from build123d import *

# Parameters (mm, degrees)
F0_W        = 11
F0_H        = 4
F0_W_2      = 10
F1_DEPTH    = 10
F2_DEPTH    = 5
F3_DEPTH    = 15
F5_DEPTH    = 40
F6_T1_DEPTH = 33.0017809158


# Not quite as in the source:
# - a fillet or chamfer that OpenCascade refuses, or shapes differently, is made with other operations: its cross-section is extruded or revolved along the edge and cut away or added


with BuildPart() as f1:
    # F0 (on Front) → F1 (new body)
    with BuildSketch(Plane.XZ):
        Polygon((-5, 4), (5, 4), (20, 4), (20, 7.5), (-20, 7.5), (-20, 4), align=None)
        with BuildLine():
            Line((-5, 0), (-5, 4))
            Line((-5, 4), (-20, 4))
            ThreePointArc((-20, 4), (-17.1715728753, 2.8284271247), (-16, 0))
            Line((-16, 0), (-5, 0))
        make_face()
        with Locations((-10.5, -2)):
            Rectangle(F0_W, F0_H)
        Polygon((16, -4), (5, -4), (-5, -4), (-16, -4), (-16, -7.5), (16, -7.5), align=None)
        with Locations((0, -2)):
            Rectangle(F0_W_2, F0_H)
        with Locations((0, 2)):
            Rectangle(F0_W_2, F0_H)
        with BuildLine():
            Line((20, 4), (5, 4))
            Line((5, 4), (5, 0))
            Line((5, 0), (16, 0))
            ThreePointArc((16, 0), (17.1715728753, 2.8284271247), (20, 4))
        make_face()
        with Locations((10.5, -2)):
            Rectangle(F0_W, F0_H)
    extrude(amount=F1_DEPTH)

    # F0 (on Front) → F2 (join)
    with BuildSketch(Plane.XZ):
        with BuildLine():
            Line((-20, 2), (-20, 4))
            ThreePointArc((-20, 4), (-24, 0), (-20, -4))
            Line((-20, -4), (-20, -2))
            ThreePointArc((-20, -2), (-22, 0), (-20, 2))
        make_face()
        with BuildLine():
            ThreePointArc((-16, 0), (-17.1715728753, 2.8284271247), (-20, 4))
            Line((-20, 4), (-20, 2))
            ThreePointArc((-20, 2), (-18.5857864376, 1.4142135624), (-18, 0))
            ThreePointArc((-18, 0), (-18.5857864376, -1.4142135624), (-20, -2))
            Line((-20, -2), (-20, -4))
            ThreePointArc((-20, -4), (-17.1715728753, -2.8284271247), (-16, 0))
        make_face()
        with BuildLine():
            Line((-16, -4), (-16, 0))
            ThreePointArc((-16, 0), (-17.1715728753, -2.8284271247), (-20, -4))
            Line((-20, -4), (-16, -4))
        make_face()
        with BuildLine():
            ThreePointArc((20, -4), (17.1715728753, -2.8284271247), (16, 0))
            Line((16, 0), (16, -4))
            Line((16, -4), (20, -4))
        make_face()
        with BuildLine():
            Line((20, 2), (20, 4))
            ThreePointArc((20, 4), (17.1715728753, 2.8284271247), (16, 0))
            ThreePointArc((16, 0), (17.1715728753, -2.8284271247), (20, -4))
            Line((20, -4), (20, -2))
            ThreePointArc((20, -2), (18, 0), (20, 2))
        make_face()
        with BuildLine():
            ThreePointArc((24, 0), (22.8284271247, 2.8284271247), (20, 4))
            Line((20, 4), (20, 2))
            ThreePointArc((20, 2), (21.4142135624, 1.4142135624), (22, 0))
            ThreePointArc((22, 0), (21.4142135624, -1.4142135624), (20, -2))
            Line((20, -2), (20, -4))
            ThreePointArc((20, -4), (22.8284271247, -2.8284271247), (24, 0))
        make_face()
    extrude(amount=F2_DEPTH)

    # F0 (on Front) → F3 (join)
    with BuildSketch(Plane.XZ):
        Polygon((16, -4), (5, -4), (-5, -4), (-16, -4), (-16, -7.5), (16, -7.5), align=None)
        with Locations((0, -2)):
            Rectangle(F0_W_2, F0_H)
        with Locations((0, 2)):
            Rectangle(F0_W_2, F0_H)
        Polygon((-5, 4), (5, 4), (20, 4), (20, 7.5), (-20, 7.5), (-20, 4), align=None)
    extrude(amount=F3_DEPTH)

    # F4 (on face) → F5 (cut)
    with BuildSketch(Plane(origin=(-20, 0, 0), x_dir=(0, -1, 0), z_dir=(-1, 0, 0))):
        with BuildLine():
            ThreePointArc((8.5, -5.75), (8.2071067812, -5.0428932188), (7.5, -4.75))
            Line((7.5, -4.75), (7.5, -6.75))
            ThreePointArc((7.5, -6.75), (8.2071067812, -6.4571067812), (8.5, -5.75))
        make_face()
        with BuildLine():
            Line((7.5, -6.75), (7.5, -4.75))
            ThreePointArc((7.5, -4.75), (6.5, -5.75), (7.5, -6.75))
        make_face()
        with BuildLine():
            ThreePointArc((7.5, 6.75), (6.5, 5.75), (7.5, 4.75))
            Line((7.5, 4.75), (7.5, 6.75))
        make_face()
        with BuildLine():
            Line((7.5, 6.75), (7.5, 4.75))
            ThreePointArc((7.5, 4.75), (8.2071067812, 5.0428932188), (8.5, 5.75))
            ThreePointArc((8.5, 5.75), (8.2071067812, 6.4571067812), (7.5, 6.75))
        make_face()
    extrude(amount=-F5_DEPTH, mode=Mode.SUBTRACT)

    # F6: chamfer of 3.5 on 2 edges, made by hand

    # F6_s2 → F6_t1 (cut)
    with BuildSketch(Plane.XZ.offset(-9.0008904579)):
        Polygon((-16, -4), (-12.5, -7.5), (-16, -7.5), align=None)
        Polygon((16, -4), (12.5, -7.5), (16, -7.5), align=None)
    extrude(amount=F6_T1_DEPTH, mode=Mode.SUBTRACT)


solid = f1.part
Input: part model. Units: mm. Frame: model coordinates. A direction names the side the tool comes from. Round coordinates to 2 decimals unless told otherwise and drop trailing zeros. Order: outer loops, then holes, each group sorted by start corner. A loop starts at its lowest first (then second) coordinate and runs counter-clockwise, first axis right, second up. Notation, with made-up numbers: (-9, 0.25) - (6, 0.25) arc R21 cw to (6, 14.25) - close; hole circle Ø3 at (-30.75, -23.5). An arc over 180 degrees is marked (long way). Answer as a JSON object with one key per item and string values. Group by question number.
(1) Cut plane C-C (z = 1). Return loops of the section in (x, y).
(2) Cut plane B-B (y = -11.5). Return loops of the section in (x, z).
(3) Reachability of faces 1 (the face through (-18, -2, -4)), 2 (the face through (-17.203, -7.465, 2.859)), 3 (the face through (18, -5, -1)), 4 (the face through (-13, -12, 4)), 5 (the face through (-20, -7, 7)) from +Z, -Z, +X, -X, +Y, -Y: full face, straight path, thin tool, end or side. Return the list, or none.
(4) Draft query along Z for faces 6 (the face through (-10, -12, -4)), 7 (the face through (15.4, -7.4, -4.6)), 8 (the face through (-16, -7, -2)). Return one class per face: released by +Z, released by -Z, zero draft, split by the parting line, or undercut.
(5) Cut plane A-A (x = 6). Return loops of the section in (y, z), then the cut area to 3 significant figures.
(6) Pin query (flat end, axial travel): P1, Ø2.5, axis at x = -20, z = 1, coming from the -Y side; P2, Ø3, axis at x = -18, y = -2.5, coming from the -Z side; P3, Ø1.8, axis at y = -6.5, z = 6, coming from the +X side. Return the tip coordinate at first contact, or that it passes through.
(7) Cut plane D-D (y = -2.5). Return loops of the section in (x, z).
(8) Material intervals for probe 1 along Z at (x, y) = (5.5, -8.25); probe 2 along Z at (x, y) = (15, -12.5); probe 3 along Z at (x, y) = (-12.5, -7), sorted ascending. Write a range as from..to.
Here are the results:
{
 "1": {"outline": "(-23.87, -5) - (-21.73, -5) - (-21.73, 0) - (-23.87, 0) - close; (-18.27, -5) - (-16.13, -5) - (-16.13, -10) - (-5, -10) - (-5, -15) - (5, -15) - (5, -10) - (16.13, -10) - (16.13, -5) - (18.27, -5) - (18.27, 0) - (-18.27, 0) - close; (21.73, -5) - (23.87, -5) - (23.87, 0) - (21.73, 0) - close"},
 "2": {"outline": "(-20, 4) - (-5, 4) - (-5, -4) - (-16, -4) - (-12.5, -7.5) - (12.5, -7.5) - (16, -4) - (5, -4) - (5, 4) - (20, 4) - (20, 7.5) - (-20, 7.5) - close"},
 "3": {"face 1": "-Z, -X, +Y, -Y", "face 2": "-Z, -X, -Y", "face 3": "-Z, +X, -Y", "face 4": "-X, -Y", "face 5": "+Z, -X, +Y, -Y"},
 "4": {"face 6": "undercut", "face 7": "released by -Z", "face 8": "zero draft"},
 "5": {"outline": "(-15, -7.5) - (0, -7.5) - (0, 7.5) - (-15, 7.5) - (-15, 4) - (-10, 4) - (-10, -4) - (-15, -4) - close; hole circle Ø2 at (-7.5, -5.75); hole circle Ø2 at (-7.5, 5.75)", "area": "179 mm^2"},
 "6": {"P1": "stops at y = -5", "P2": "stops at z = -4", "P3": "stops at x = 20"},
 "7": {"outline": "(-20, -4) - (-16, -4) - (-12.5, -7.5) - (12.5, -7.5) - (16, -4) - (20, -4) arc R4 ccw to (20, 4) - (20, 7.5) - (-20, 7.5) - (-20, 4) arc R4 ccw to start; hole circle Ø4 at (-20, 0); hole circle Ø4 at (20, 0)"},
 "8": {"probe 1": "z = -7.5..-6.41, -5.09..5.09, 6.41..7.5", "probe 2": "z = -5..-4, 4..7.5", "probe 3": "z = -7.5..-6.62, -4.88..4.88, 6.62..7.5"}
}
